```python
from build123d import *

# Parameters (mm, degrees)
F0_W     = 11
F0_H     = 30
F1_DEPTH = 24
F3_DEPTH = 25
F4_R     = 5
F4_R_2   = 2.5
F5_DEPTH = 25
F6_R     = 13
F7_R     = 5
F8_R     = 2


with BuildPart() as f1:
    # F0 (on Front) → F1 (new body, symmetric)
    with BuildSketch(Plane.XZ):
        with BuildLine():
            ThreePointArc((-27.6980438828, -19.9313075026), (-27.1710581859, -14.3329659721), (-25.6086153568, -8.9313075026))
            Line((-25.6086153568, -8.9313075026), (-53.6980438828, -8.9313075026))
            Line((-53.6980438828, -8.9313075026), (-53.6980438828, -19.9313075026))
            Line((-53.6980438828, -19.9313075026), (-27.6980438828, -19.9313075026))
        make_face()
        with BuildLine():
            Line((-13.1899772677, -8.9313075026), (-25.6086153568, -8.9313075026))
            ThreePointArc((-25.6086153568, -8.9313075026), (-27.1710581859, -14.3329659721), (-27.6980438828, -19.9313075026))
            Line((-27.6980438828, -19.9313075026), (-16.6980438828, -19.9313075026))
            ThreePointArc((-16.6980438828, -19.9313075026), (-15.7997942721, -14.1583851192), (-13.1899772677, -8.9313075026))
        make_face()
        with BuildLine():
            Line((17.793889502, -8.9313075026), (30.2125275911, -8.9313075026))
            ThreePointArc((30.2125275911, -8.9313075026), (2.3019561172, 10.0686924974), (-25.6086153568, -8.9313075026))
            Line((-25.6086153568, -8.9313075026), (-13.1899772677, -8.9313075026))
            ThreePointArc((-13.1899772677, -8.9313075026), (2.3019561172, -0.9313075026), (17.793889502, -8.9313075026))
        make_face()
        with BuildLine():
            ThreePointArc((32.3019561172, -19.9313075026), (31.7749704202, -14.3329659721), (30.2125275911, -8.9313075026))
            Line((30.2125275911, -8.9313075026), (17.793889502, -8.9313075026))
            ThreePointArc((17.793889502, -8.9313075026), (20.4037065064, -14.1583851192), (21.3019561172, -19.9313075026))
            Line((21.3019561172, -19.9313075026), (32.3019561172, -19.9313075026))
        make_face()
        with BuildLine():
            Line((53.3019561172, -8.9313075026), (42.3019561172, -8.9313075026))
            Line((42.3019561172, -8.9313075026), (30.2125275911, -8.9313075026))
            ThreePointArc((30.2125275911, -8.9313075026), (31.7749704202, -14.3329659721), (32.3019561172, -19.9313075026))
            Line((32.3019561172, -19.9313075026), (53.3019561172, -19.9313075026))
            Line((53.3019561172, -19.9313075026), (53.3019561172, -8.9313075026))
        make_face()
        with Locations((47.8019561172, 6.0686924974)):
            Rectangle(F0_W, F0_H)
    extrude(amount=F1_DEPTH, both=True)

    # F2 (on face) → F3 (cut)
    with BuildSketch(Plane.YZ.offset(53.3019561172)):
        with BuildLine():
            ThreePointArc((-6.5, 5.0686926821), (-9.23e-08, -1.4313075026), (6.5, 5.0686924974))
            ThreePointArc((6.5, 5.0686924974), (9.23e-08, 11.5686924974), (-6.5, 5.0686926821))
        make_face()
        with BuildLine():
            ThreePointArc((-6.5, 5.0686926821), (9.23e-08, 11.5686924974), (6.5, 5.0686924974))
            Line((6.5, 5.0686924974), (6.5, 21.0686924974))
            Line((6.5, 21.0686924974), (-6.5, 21.0686924974))
            Line((-6.5, 21.0686924974), (-6.5, 5.0686926821))
        make_face()
    extrude(amount=-F3_DEPTH, mode=Mode.SUBTRACT)

    # F4 (on face) → F5 (cut, symmetric)
    with BuildSketch(Plane.XY.offset(-8.9313075026)):
        with Locations((-39.6533296198, -11)):
            Circle(F4_R)
        with Locations((-39.6533296198, 11)):
            Circle(F4_R)
        Circle(F4_R_2)
    extrude(amount=F5_DEPTH, both=True, mode=Mode.SUBTRACT)

    # F6
    f6_edges = [f1.edges().sort_by_distance(p)[0] for p in [
        (-53.698044, 24, -14.431308),
        (-53.698044, -24, -14.431308),
    ]]
    fillet(f6_edges, radius=F6_R)

    # F7
    f7_edges = [f1.edges().sort_by_distance(p)[0] for p in [
        (47.801956, 24, 21.068692),
        (47.801956, -24, 21.068692),
    ]]
    fillet(f7_edges, radius=F7_R)

    # F8
    f8_edges = [f1.edges().sort_by_distance(p)[0] for p in [
        (30.212528, 0, -8.931308),
        (-25.608615, 0, -8.931308),
    ]]
    fillet(f8_edges, radius=F8_R)


solid = f1.part
```
Verification items for the finished model (mm, model axes). A direction names the side the tool comes from. Coordinates: 2 decimals unless noted, no trailing zeros. Loops run counter-clockwise (first coordinate to the right, second up) from the corner with the lowest first, then second, coordinate; pieces in that order, holes last. Notation, with made-up numbers: (83.5, 83) -> (136.5, 83) arc R21 cw to (136.5, 100) -> close; hole circle Ø4 at (65.25, -39). An arc over 180 degrees is marked (long way). Answer in a Markdown table with one row per item. Add a question column.
1. Section check A-A, the plane z = -13.5. Enter the section's corners in (x, y).
2. Material ranges on probe 1 along X at (y, z) = (-12, -13); probe 2 along X at (y, z) = (14, -10); probe 3 along Y at (x, z) = (46, 15.5), recorded low to high. Write a range as [from, to].
3. Draft check along Y on faces 4 (the face through (47.88, -0.14, -1.43)), 5 (the face through (48, 13, 21.069)), 6 (the face through (47.88, 22.57, 19.57)). Enter one of: +Y half, -Y half, draft (parallel to the pull), parting line (faces both ways), or undercut.
4. Access from +Z, -Z, +X, -X, +Y, -Y to the whole of each face (thin tool, end or side, straight path). Record for faces 1 (the face through (37, 0, -8.931)), 2 (the face through (-40, 0, -8.931)), 3 (the face through (48, -6.5, 13)).
5. Depth check by flat-ended pin: P1, Ø21.5, axis at x = -38.5, y = 2.5, coming from the +Z side; P2, Ø4, axis at y = -9.5, z = 17, coming from the -X side; P3, Ø5, axis at x = 38, z = 4.5, coming from the -Y side; P4, Ø1.5, axis at x = 15.5, y = -6, coming from the +Z side. Enter the tip coordinate at first touch or a pass-through.
6. Section check D-D, the plane z = 13. Enter the section's corners in (x, y), then the cut area to 3 significant figures.
7. Section check C-C, the plane x = 0. Enter the section's corners in (y, z), then the cut area to 3 significant figures.
8. Section check B-B, the plane y = 12. Enter the section's corners in (x, z), then the cut area to 3 significant figures.
Derived:
| question | item | result |
|---|---|---|
| 1 | outline | (-53.7, -11) arc R13 ccw to (-40.7, -24) -> (-15.58, -24) -> (-15.58, 24) -> (-40.7, 24) arc R13 ccw to (-53.7, 11) -> close; (20.18, -24) -> (53.3, -24) -> (53.3, 24) -> (20.18, 24) -> close; hole circle Ø10 at (-39.65, -11); hole circle Ø10 at (-39.65, 11) |
| 2 | probe 1 | x = [-53.66, -44.55], [-34.75, -15.39], [19.99, 53.3] |
| 2 | probe 2 | x = [-53.35, -43.65], [-35.65, -13.9], [18.5, 53.3] |
| 2 | probe 3 | y = [-24, -6.5], [6.5, 24] |
| 3 | face 4 | undercut |
| 3 | face 5 | draft |
| 3 | face 6 | +Y half |
| 4 | face 1 | +Z, +Y, -Y |
| 4 | face 2 | +Z, -X, +Y, -Y |
| 4 | face 3 | +Z, +X |
| 5 | P1 | stops at z = -8.93 |
| 5 | P2 | stops at x = 42.3 |
| 5 | P3 | passes through |
| 5 | P4 | stops at z = 7.36 |
| 6 | outline | (42.3, -24) -> (53.3, -24) -> (53.3, -6.5) -> (42.3, -6.5) -> close; (42.3, 6.5) -> (53.3, 6.5) -> (53.3, 24) -> (42.3, 24) -> close |
| 6 | area | 385 mm² |
| 7 | outline | (-24, -1.07) -> (-2.5, -1.07) -> (-2.5, 9.98) -> (-24, 9.98) -> close; (2.5, -1.07) -> (24, -1.07) -> (24, 9.98) -> (2.5, 9.98) -> close |
| 7 | area | 475 mm² |
| 8 | outline | (-53.66, -19.93) -> (-44.55, -19.93) -> (-44.55, -8.93) -> (-53.66, -8.93) -> close; (-34.75, -19.93) -> (-16.7, -19.93) arc R19 cw to (21.3, -19.93) -> (53.3, -19.93) -> (53.3, 21.07) -> (42.3, 21.07) -> (42.3, -8.93) -> (31.54, -8.93) arc R2 cw to (29.71, -7.74) arc R30 ccw to (-25.11, -7.74) arc R2 cw to (-26.94, -8.93) -> (-34.75, -8.93) -> close |
| 8 | area | 1,600 mm² |
